Verification items for the finished model (mm, model axes). Face numbers are marked on the shaded views. A direction names the side the tool comes from. Coordinates: 2 decimals unless noted, no trailing zeros. Order: outer loops, then holes, each group sorted by start corner. A loop starts at its lowest first (then second) coordinate and runs counter-clockwise, first axis right, second up. Notation, with made-up numbers: (-27.5, 57.5) - (-9.5, 57.5) arc R9 ccw to (-9.5, 71.5) - close; hole circle Ø4 at (-15.5, 6.5). An arc over 180 degrees is marked (long way). Answer as CSV lines item,"result". Start each with the question number.
1. Mould release check, pull along Y, two halves, no side actions. Record for the marked faces 5, 6, 7 and 8: pulls with the +Y half, pulls with the -Y half, needs draft (parallel to the pull), parting line crosses it, or undercut.
2. Section check A-A (x = 0). Record the cut outline in (y, z).
3. Material ranges on L1, parallel to Y at x = -7.9, z = 0; L2, parallel to Z at x = -8.3, y = 4.9; L3, parallel to Z at x = -2, y = 20.3, recorded low to high. Write a range as [from, to].
4. Set-up check for the marked faces 1, 2, 3 and 4: record each of +Z, -Z, +X, -X, +Y, -Y from which the full face is reachable in a straight line by a thin tool's end or side.
5. Section check C-C (y = 31). Record the cut outline in (x, z).
6. Section check B-B (y = 5.5). Record the cut outline in (x, z), and give its area (3 significant figures).
7. Section check D-D (y = 18). Record the cut outline in (x, z), and give its area (3 significant figures).
8. Go/stop test with flat-tipped pins: pin 1 (6 mm diameter, centred on y = 26.5, z = -3, fed in from -X); pin 2 (2.5 mm diameter, centred on y = 20.3, z = 0, fed in from -X); pin 3 (1.5 mm diameter, centred on y = 19.5, z = 0.5, fed in from +X). Record where each tip stops, or that it passes through.
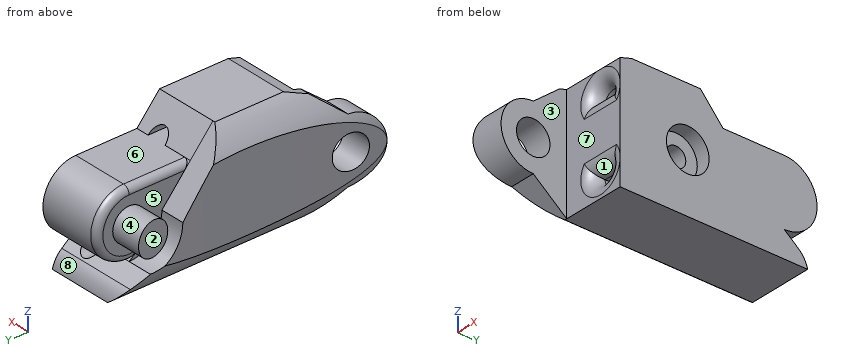
from build123d import *

# Parameters (mm, degrees)
BOSS_EXTRUDE1_DEPTH      = 40
CUT_EXTRUDE1_DEPTH       = 58
CUT_EXTRUDE2_REACH       = 47.222
SKETCH3_W                = 12
SKETCH3_H                = 10
SKETCH4_R                = 2.55
CUT_EXTRUDE3_DEPTH       = 17.5
FILLET4_R                = 2
CUT_EXTRUDE5_START       = -12.324555
SKETCH6_R                = 2.5
CUT_EXTRUDE5_DEPTH       = 9.6
CUT_EXTRUDE6_START       = 6.279445
SKETCH6_3_R              = 2.5
CUT_EXTRUDE6_DEPTH       = 6.604
CUT_EXTRUDE7_START       = -14.986
CUT_EXTRUDE7_DEPTH       = 14.986
CUT_EXTRUDE14_DEPTH      = 10
CUT_EXTRUDE14_DEPTH_BACK = 20
FILLET3_R                = 1
CUT_EXTRUDE17_DEPTH      = 9
CUT_EXTRUDE17_DEPTH_BACK = 31
SKETCH19_W               = 18.14397799
SKETCH19_H               = 52.511082079
SKETCH20_R               = 3.25
CUT_EXTRUDE18_DEPTH      = 2.1
SKETCH21_R               = 1.5
CUT_EXTRUDE19_DEPTH      = 9.1
CUT_EXTRUDE20_DEPTH      = 14
CUT_EXTRUDE20_DEPTH_BACK = 14


with BuildPart() as part:
    # Sketch1 → Boss-Extrude1 (new body)
    with BuildSketch(Plane(origin=(0, 0, 0), x_dir=(1, 0, 0), z_dir=(0, 1, 0))):
        with BuildLine():
            Line((-6.32455532, 9), (6.32455532, 9))
            ThreePointArc((6.32455532, 9), (11, 0), (6.32455532, -9))
            Line((6.32455532, -9), (-6.32455532, -9))
            ThreePointArc((-6.32455532, -9), (-11, 0), (-6.32455532, 9))
        make_face()
    extrude(amount=BOSS_EXTRUDE1_DEPTH)

    # Sketch2 → Cut-Extrude1 (cut)
    with BuildSketch(Plane.XZ):
        with BuildLine():
            Line((1.5, 5), (-1.5, 5))
            ThreePointArc((-1.5, 5), (0, 6.5), (1.5, 5))
        make_face()
        with BuildLine():
            Line((1.5, -5), (-1.5, -5))
            ThreePointArc((-1.5, -5), (0, -6.5), (1.5, -5))
        make_face()
    extrude(amount=-CUT_EXTRUDE1_DEPTH, mode=Mode.SUBTRACT)

    # Cut-Extrude2: up to this face of the body (flat: up to its plane)
    cut_extrude2_end = Plane(part.part.faces().sort_by_distance((0, 20, 9))[0])
    # Sketch3 → Cut-Extrude2 (cut, up to the picked face)
    with BuildSketch(Plane(origin=(0, 0, -9), x_dir=(-1, 0, 0), z_dir=(0, 0, -1)), mode=Mode.PRIVATE) as cut_extrude2_sk1:
        with Locations((0, 5)):
            Rectangle(SKETCH3_W, SKETCH3_H)
    cut_extrude2_tool1 = split(extrude(cut_extrude2_sk1.sketch, amount=-CUT_EXTRUDE2_REACH, mode=Mode.PRIVATE), bisect_by=cut_extrude2_end, keep=Keep.BOTH, mode=Mode.PRIVATE)
    add(cut_extrude2_tool1.solids().sort_by(Axis((0, 5, -9), (0, 0, 1)))[0], mode=Mode.SUBTRACT)

    # Sketch4 → Cut-Extrude3 (cut, symmetric)
    with BuildSketch(Plane.ZY.offset(-6)):
        with Locations(Location((0, 4.9, 0), (0, 0, 270))):
            Circle(SKETCH4_R)
        with BuildLine():
            Line((-9, 10), (-4.9, 4.9))
            ThreePointArc((-4.9, 4.9), (0, 0), (4.9, 4.9))
            Line((4.9, 4.9), (9, 10))
            Line((9, 10), (12.043777938, -1.930413563))
            Line((12.043777938, -1.930413563), (-10.290438773, -1.930413563))
            Line((-10.290438773, -1.930413563), (-9, 10))
        make_face()
    extrude(amount=CUT_EXTRUDE3_DEPTH, both=True, mode=Mode.SUBTRACT)

    # Fillet4
    fillet4_edges = [part.edges().sort_by_distance(p)[0] for p in [
        (0, 10, 5),
        (0, 10, 6.5),
        (0, 10, -5),
        (0, 10, -6.5),
    ]]
    fillet(fillet4_edges, radius=FILLET4_R)

    # Sketch6 → Cut-Extrude5 (cut)
    with BuildSketch(Plane.ZY.offset(6.32455532).offset(CUT_EXTRUDE5_START)):
        with BuildLine():
            Line((9, 22.232353468), (0, 30))
            ThreePointArc((0, 30), (-3.535533906, 31.464466094), (-5, 35))
            Line((-5, 35), (-6.715621335, 37.134065563))
            ThreePointArc((-6.715621335, 37.134065563), (-7.737273484, 38.043034193), (-9, 38.567933069))
            Line((-9, 38.567933069), (-20.985236203, 70.297327945))
            Line((-20.985236203, 70.297327945), (29.827478779, 37.594689174))
            Line((29.827478779, 37.594689174), (9, 22.232353468))
        make_face()
        with Locations((0, 35)):
            Circle(SKETCH6_R, mode=Mode.SUBTRACT)
    extrude(amount=-CUT_EXTRUDE5_DEPTH, mode=Mode.SUBTRACT)

    # Sketch6<3> → Cut-Extrude6 (cut)
    with BuildSketch(Plane.ZY.offset(6.32455532).offset(CUT_EXTRUDE6_START)):
        with BuildLine():
            Line((9, 22.232353468), (0, 30))
            ThreePointArc((0, 30), (-3.535533906, 31.464466094), (-5, 35))
            Line((-5, 35), (-6.715621335, 37.134065563))
            ThreePointArc((-6.715621335, 37.134065563), (-7.737273484, 38.043034193), (-9, 38.567933069))
            Line((-9, 38.567933069), (-20.985236203, 70.297327945))
            Line((-20.985236203, 70.297327945), (29.827478779, 37.594689174))
            Line((29.827478779, 37.594689174), (9, 22.232353468))
        make_face()
        with Locations((0, 35)):
            Circle(SKETCH6_3_R, mode=Mode.SUBTRACT)
    extrude(amount=-CUT_EXTRUDE6_DEPTH, mode=Mode.SUBTRACT)

    # Sketch7 → Cut-Extrude7 (cut)
    with BuildSketch(Plane(origin=(6, 0, 0), x_dir=(0, 0, -1), z_dir=(1, 0, 0)).offset(CUT_EXTRUDE7_START)):
        with BuildLine():
            Line((5, 35), (6.715621335, 37.134065563))
            ThreePointArc((6.715621335, 37.134065563), (7.737273484, 38.043034193), (9, 38.567933069))
            Line((9, 38.567933069), (57.758012517, 25.684640815))
            Line((57.758012517, 25.684640815), (-30.579133969, 55.486762513))
            Line((-30.579133969, 55.486762513), (-9, 22.232353468))
            Line((-9, 22.232353468), (-5, 25.684640815))
            Line((-5, 25.684640815), (-5, 35))
            ThreePointArc((-5, 35), (0, 40), (5, 35))
        make_face()
    extrude(amount=CUT_EXTRUDE7_DEPTH, mode=Mode.SUBTRACT)

    # Sketch16 → Cut-Extrude14 (cut, two sides: drawn at the far end of the back side and taken through both)
    with BuildSketch(Plane.ZY.offset(6.32455532).offset(-CUT_EXTRUDE14_DEPTH_BACK)):
        Polygon((8.113259987, 8.896981935), (11.550119513, 20.031417135), (18.056002312, 15.695207893), (16.156055326, 2.281594324), align=None)
    extrude(amount=CUT_EXTRUDE14_DEPTH + CUT_EXTRUDE14_DEPTH_BACK, mode=Mode.SUBTRACT)

    # Fillet3
    # the kernel refuses this fillet: 1 mm, written as the material it takes off along each edge
    with BuildSketch(Plane(origin=(5.99999968, 23.184640014, 5), x_dir=(-1, 0, 0), z_dir=(0, 1, 0))) as fillet3_piece_1_section:
        with BuildLine():
            CenterArc((FILLET3_R, -FILLET3_R), FILLET3_R, 90, 90)
            Line((0, -FILLET3_R), (0, 0))
            Line((0, 0), (FILLET3_R, 0))
        make_face()
    fillet3_piece_1 = extrude(amount=11.815359986, mode=Mode.PRIVATE)
    fillet3_piece_1 = split(fillet3_piece_1, bisect_by=Plane(origin=(5.764976342, 27.542151825, 2.84779096), z_dir=(0, 0.7570343753275034, 0.653375048936288)), keep=Keep.TOP, mode=Mode.PRIVATE)
    add(fillet3_piece_1, mode=Mode.SUBTRACT)
    with BuildSketch(Plane(origin=(6, 35, 0), x_dir=(0, 0, 1), z_dir=(0, -1, 0))) as fillet3_piece_2_section:
        with BuildLine():
            CenterArc((4, 1.00000032), FILLET3_R, 270, 90)
            ThreePointArc((4, 3.2e-07), (4.5, 3.2e-07), (5, 0))
            Line((5, 0), (5, 1.00000032))
        make_face()
    fillet3_piece_2 = revolve(axis=Axis((6, 35, 0), (-1, 0, 0)), revolution_arc=208.693968336, mode=Mode.PRIVATE)
    fillet3_piece_2 = split(fillet3_piece_2, bisect_by=Plane(origin=(5.717618036, 35.865387036, -5.695703303), z_dir=(0, 0.6265569118246592, 0.7793756708062848)), keep=Keep.TOP, mode=Mode.PRIVATE)
    add(fillet3_piece_2, mode=Mode.SUBTRACT)
    with BuildSketch(Plane(origin=(-6.00000032, 35, 0), x_dir=(0, -0.48013104288571373, -0.8771967747646344), z_dir=(0, -0.8771967747646344, 0.48013104288571373))) as fillet3_piece_3_section:
        with BuildLine():
            CenterArc((5 - FILLET3_R, FILLET3_R), FILLET3_R, 270, 90)
            Line((5 - FILLET3_R, 0), (5, 0))
            Line((5, 0), (5, FILLET3_R))
        make_face()
    fillet3_piece_3 = revolve(axis=Axis((-6.00000032, 35, 0), (1, 0, 0)), revolution_arc=208.69396098, mode=Mode.PRIVATE)
    fillet3_piece_3 = split(fillet3_piece_3, bisect_by=Plane(origin=(-5.717618693, 35.865387047, -5.695703312), z_dir=(0, 0.6265569118246592, 0.7793756708062848)), keep=Keep.TOP, mode=Mode.PRIVATE)
    add(fillet3_piece_3, mode=Mode.SUBTRACT)
    with BuildSketch(Plane(origin=(-6.00000032, 35, 5), x_dir=(0, 0, -1), z_dir=(0, -1, 0))) as fillet3_piece_4_section:
        with BuildLine():
            CenterArc((FILLET3_R, FILLET3_R), FILLET3_R, 180, 90)
            Line((0, FILLET3_R), (0, 0))
            Line((0, 0), (FILLET3_R, 0))
        make_face()
    fillet3_piece_4 = extrude(amount=11.815359185, mode=Mode.PRIVATE)
    fillet3_piece_4 = split(fillet3_piece_4, bisect_by=Plane(origin=(-5.831638777, 29.468233552, 0.616132314), z_dir=(0, 0.7570343753275034, 0.653375048936288)), keep=Keep.TOP, mode=Mode.PRIVATE)
    add(fillet3_piece_4, mode=Mode.SUBTRACT)

    # Sketch19 → Cut-Extrude17 (cut, two sides: drawn at the far end of the back side and taken through both)
    with BuildSketch(Plane.XY.offset(5).offset(-CUT_EXTRUDE17_DEPTH_BACK)):
        with Locations((12.571988995, 20.723484304)):
            Rectangle(SKETCH19_W, SKETCH19_H)
    extrude(amount=CUT_EXTRUDE17_DEPTH + CUT_EXTRUDE17_DEPTH_BACK, mode=Mode.SUBTRACT)

    # Sketch20 → Cut-Extrude18 (cut)
    with BuildSketch(Plane(origin=(3.5, 0, 0), x_dir=(0, 0, -1), z_dir=(1, 0, 0))):
        with Locations(Location((0, 20.3, 0), (0, 0, 90))):
            Circle(SKETCH20_R)
    extrude(amount=-CUT_EXTRUDE18_DEPTH, mode=Mode.SUBTRACT)

    # Sketch21 → Cut-Extrude19 (cut)
    with BuildSketch(Plane(origin=(1.4, 0, 0), x_dir=(0, 0, -1), z_dir=(1, 0, 0))):
        with Locations(Location((0, 20.3, 0), (0, 0, 90))):
            Circle(SKETCH21_R)
    extrude(amount=-CUT_EXTRUDE19_DEPTH, mode=Mode.SUBTRACT)

    # Sketch17 → Cut-Extrude20 (cut, two sides: drawn at the far end of the back side and taken through both)
    with BuildSketch(Plane.XY.offset(-CUT_EXTRUDE20_DEPTH_BACK)):
        with BuildLine():
            Line((11, 0), (21.82042967, 52.006672347))
            Line((21.82042967, 52.006672347), (-19.981455648, 54.836748038))
            Line((-19.981455648, 54.836748038), (-22.103338511, 10.056999989))
            Line((-22.103338511, 10.056999989), (-11, 0))
            ThreePointArc((-11, 0), (-9.292734081, 20), (-11, 40))
            Line((-11, 40), (-14.776436098, 42.476608752))
            Line((-14.776436098, 42.476608752), (-7.177261686, 49.84322342))
            Line((-7.177261686, 49.84322342), (9.09969288, 46.456664847))
            Line((9.09969288, 46.456664847), (16.101427872, 37.54860329))
            Line((16.101427872, 37.54860329), (11, 40))
            ThreePointArc((11, 40), (9.292734081, 20), (11, 0))
        make_face()
    extrude(amount=CUT_EXTRUDE20_DEPTH + CUT_EXTRUDE20_DEPTH_BACK, mode=Mode.SUBTRACT)


solid = part.part
Evaluation:
1,face 5,"undercut"
1,face 6,"needs draft"
1,face 7,"pulls with the -Y half"
1,face 8,"pulls with the +Y half"
2,outline,"(10, -9) - (38.57, -9) arc R4.12 ccw to (37.13, -6.72) - (36.87, -6.5) - (12, -6.5) arc R2 ccw to (10, -8.5) - close; (10, -3) arc R2 ccw to (12, -5) - (35, -5) arc R5 ccw to (35, 5) - (12, 5) arc R2 ccw to (10, 3) - close; (10, 8.45) arc R2 ccw to (12, 6.5) - (24.39, 6.5) - (22.23, 9) - (11.77, 9) - close; hole circle Ø3 at (20.3, 0)"
3,L1,"y = [0, 2.35], [7.45, 30], [32.5, 37.5]"
3,L2,"z = [-4.9, -2.55], [2.55, 4.9]"
3,L3,"z = [-9, -1.5], [1.5, 9]"
4,face 1,"-Y"
4,face 2,"+Z, -Z, -X"
4,face 3,"+Z, -Z, +X, -Y"
4,face 4,"-X"
5,outline,"(-9.81, -4.98) arc R11 ccw to (-6.32, -9) - (3.5, -9) - (3.5, 5) - (-5, 5) arc R1 ccw to (-6, 4) - (-6, -3) - (-9.81, -3) - close; hole (-1.5, -5) arc R1.5 ccw to (1.5, -5) - close"
6,outline,"(-10.19, -4.15) arc R11 ccw to (-9.59, -5.38) - (-6, -5.38) - (-6, -2.48) - (-10.19, -2.48) - close; (-10.19, 2.48) - (-6, 2.48) - (-6, 5.38) - (-9.59, 5.38) arc R11 ccw to (-10.19, 4.15) - close"
6,area,"23.6 mm²"
7,outline,"(-9.31, -5.86) arc R11 ccw to (-6.32, -9) - (3.5, -9) - (3.5, -2.3) - (1.4, -2.3) - (1.4, 2.3) - (3.5, 2.3) - (3.5, 9) - (-6.32, 9) arc R11 ccw to (-9.31, 5.86) - close; hole (-1.5, -5) arc R1.5 ccw to (1.5, -5) - close; hole (-1.5, 5) - (1.5, 5) arc R1.5 ccw to start"
7,area,"206 mm²"
8,pin 1,"stops at x = -9.68"
8,pin 2,"stops at x = -9.3"
8,pin 3,"stops at x = 1.4"
